CAD build for the part. Positions are in the model's coordinates, mm. A direction names the side the tool comes from. Round coordinates to 2 decimals unless told otherwise and drop trailing zeros. Order: outer loops, then holes, each group sorted by start corner. A loop starts at its lowest first (then second) coordinate and runs counter-clockwise, first axis right, second up. Notation, with made-up numbers: M 8.5,-17 L 40.5,-17 A15 ccw 40.5,7 Z; hole C 62.5,25 d2. An arc over 180 degrees is marked long. Answer as a JSON object with one key per item and string values.
```python
from build123d import *

# Parameters (mm, degrees)
SKETCH_1_R               = 7.5
EXTRUDE_1_DEPTH          = 10
SKETCH_2_W               = 20
SKETCH_2_H               = 20
EXTRUDE_2_DEPTH          = 24
SKETCH_3_W               = 68
SKETCH_3_H               = 68
EXTRUDE_3_DEPTH          = 8
FILLET_1_R               = 10
SKETCH_4_R               = 2
CUT_EXTRUDE_1_DEPTH      = 23
PATTERN_CIRCULAR_1_COUNT = 2
PATTERN_CIRCULAR_1_ANGLE = 90
SKETCH_5_R               = 5
CUT_EXTRUDE_2_DEPTH      = 31
FILLET_3_R               = 4
SKETCH_6_W               = 15.6
SKETCH_6_H               = 15.6
CUT_EXTRUDE_3_DEPTH      = 3
SKETCH_7_R               = 3
EXTRUDE_4_DEPTH          = 12
FILLET_4_R               = 2


with BuildPart() as part:
    # 草图1 → 凸台-拉伸1 (new body)
    with BuildSketch(Plane(origin=(0, 0, 0), x_dir=(1, 0, 0), z_dir=(0, 1, 0))):
        with Locations(Location((0, 0, 0), (0, 0, 270))):
            Circle(SKETCH_1_R)
    extrude(amount=EXTRUDE_1_DEPTH)

    # 草图2 → 凸台-拉伸2 (add)
    with BuildSketch(Plane.XZ):
        Rectangle(SKETCH_2_W, SKETCH_2_H)
    extrude(amount=EXTRUDE_2_DEPTH)

    # 草图3 → 凸台-拉伸3 (add)
    with BuildSketch(Plane.XZ.offset(24)):
        Rectangle(SKETCH_3_W, SKETCH_3_H)
    extrude(amount=EXTRUDE_3_DEPTH)

    # 圆角1
    fillet_1_edges = [part.edges().sort_by_distance(p)[0] for p in [
        (34, -28, -34),
        (34, -28, 34),
        (-34, -28, 34),
        (-34, -28, -34),
    ]]
    fillet(fillet_1_edges, radius=FILLET_1_R)

    # 草图4 → 切除-拉伸1 (cut)
    with BuildSketch(Plane(origin=(10, 0, 0), x_dir=(0, 0, -1), z_dir=(1, 0, 0))):
        with Locations((0, -4)):
            Circle(SKETCH_4_R)
        with Locations((0, -12)):
            Circle(SKETCH_4_R)
    cut_extrude_1 = extrude(amount=-CUT_EXTRUDE_1_DEPTH, mode=Mode.SUBTRACT)

    # 阵列(圆周)1: 切除-拉伸1 ×2 about axis
    pattern_circular_1_axis = Axis((0, 10, 0), (0, -1, 0))
    for i in range(1, PATTERN_CIRCULAR_1_COUNT):
        add(cut_extrude_1.rotate(pattern_circular_1_axis, i * PATTERN_CIRCULAR_1_ANGLE / (PATTERN_CIRCULAR_1_COUNT - 1)), mode=Mode.SUBTRACT)

    # 草图5 → 切除-拉伸2 (cut)
    with BuildSketch(Plane.XZ.offset(32)):
        with Locations(Location((0, 0, 0), (0, 0, 270))):
            Circle(SKETCH_5_R)
    extrude(amount=-CUT_EXTRUDE_2_DEPTH, mode=Mode.SUBTRACT)

    # 圆角3
    fillet_3_edges = [part.edges().sort_by_distance(p)[0] for p in [
        (10, -24, 0),
        (0, -24, 10),
        (-10, -24, 0),
        (0, -24, -10),
    ]]
    fillet(fillet_3_edges, radius=FILLET_3_R)

    # 草图6 → 切除-拉伸3 (cut)
    with BuildSketch(Plane(origin=(0, -24, 0), x_dir=(1, 0, 0), z_dir=(0, 1, 0))):
        with Locations((0, -22.2)):
            Rectangle(SKETCH_6_W, SKETCH_6_H)
    extrude(amount=-CUT_EXTRUDE_3_DEPTH, mode=Mode.SUBTRACT)

    # 草图7 → 凸台-拉伸4 (add)
    with BuildSketch(Plane(origin=(0, 10, 0), x_dir=(1, 0, 0), z_dir=(0, 1, 0))):
        with Locations(Location((0, 0, 0), (0, 0, 270))):
            Circle(SKETCH_7_R)
    extrude(amount=EXTRUDE_4_DEPTH)

    # 圆角4
    fillet_4_edges = [part.edges().sort_by_distance(p)[0] for p in [
        (0, 0, -7.5),
    ]]
    fillet(fillet_4_edges, radius=FILLET_4_R)


solid = part.part
```
Item 1: Saw through at B-B on y = -25. List the corners of the cut face in (x, z).
Worked answers:
{"outline": "M -34,-24 A10 ccw -24,-34 L 24,-34 A10 ccw 34,-24 L 34,24 A10 ccw 24,34 L -24,34 A10 ccw -34,24 Z; hole M -7.8,14.4 L 7.8,14.4 L 7.8,30 L -7.8,30 Z; hole C 0,0 d10"}
Item 2: Saw through at A-A on y = -4. List the corners of the cut face in (x, z).
Worked answers:
{"outline": "M -10,-10 L -2,-10 L -2,-4.58 A5 cw -4.58,-2 L -10,-2 Z; M -10,2 L -4.58,2 A5 cw -2,4.58 L -2,10 L -10,10 Z; M 2,-10 L 10,-10 L 10,-2 L 4.58,-2 A5 cw 2,-4.58 Z; M 2,4.58 A5 cw 4.58,2 L 10,2 L 10,10 L 2,10 Z"}
Item 3: 3-axis set-ups, long thin cutter, end or side, ignore diameter. For faces 1 (the flat face through (0, -25, 30)), 2 (the flat face through (-2, -10, -10)), 3 (the flat face through (0, -1, 0)): which of +Z, -Z, +X, -X, +Y, -Y reach the whole face in a straight line?
Worked answers:
{"face 1": "+Y", "face 2": "-Z, +X, -X, +Y", "face 3": "-Y"}
Item 4: Drop flat-ended pins along their axis: pin 1 Ø4 at (x, z) = (4.5, 27) entering from +Y; pin 2 Ø6 at (x, y) = (-1.5, -9) entering from +Z; pin 3 Ø6 at (y, z) = (-5.5, 4) entering from +X; pin 4 Ø2.5 at (x, y) = (0, -12) entering from +Z. Give the stop position or say it passes through.
Worked answers:
{"pin 1": "stops at y = -27", "pin 2": "stops at z = 10", "pin 3": "stops at x = 10", "pin 4": "passes through"}
Item 5: Wall check: line 1 along Y through (x, z) = (6.2, 0); line 2 along X through (y, z) = (-19.5, 0); line 3 along Z through (x, y) = (-2, -24.5). Give the ranges that are in metal, low to high. Write a range as [from, to].
Worked answers:
{"line 1": "y = [-32, -14], [-10, -6], [-2, 10]", "line 2": "x = [-10, -5], [5, 10]", "line 3": "z = [-34, -4.58], [4.58, 14.4], [30, 34]"}
Item 6: Two-plate mould, pull along Y, no slides. Class faces 4 (the flat face through (-34, -28, 0)), 5 (the cylindrical face through (-7, -12, 2)), 6 (the cylindrical face through (11.203, -22.859, 0.196)): released by +Y, released by -Y, zero draft, split by the parting line, or undercut.
Worked answers:
{"face 4": "zero draft", "face 5": "undercut", "face 6": "released by +Y"}
Item 7: Saw through at C-C on z = 0. State how many separate pieces and enclosed holes the cut face has, and give its area (3 significant figures).
Worked answers:
{"separate pieces": "5", "enclosed holes": "0", "area": "865 mm2"}
